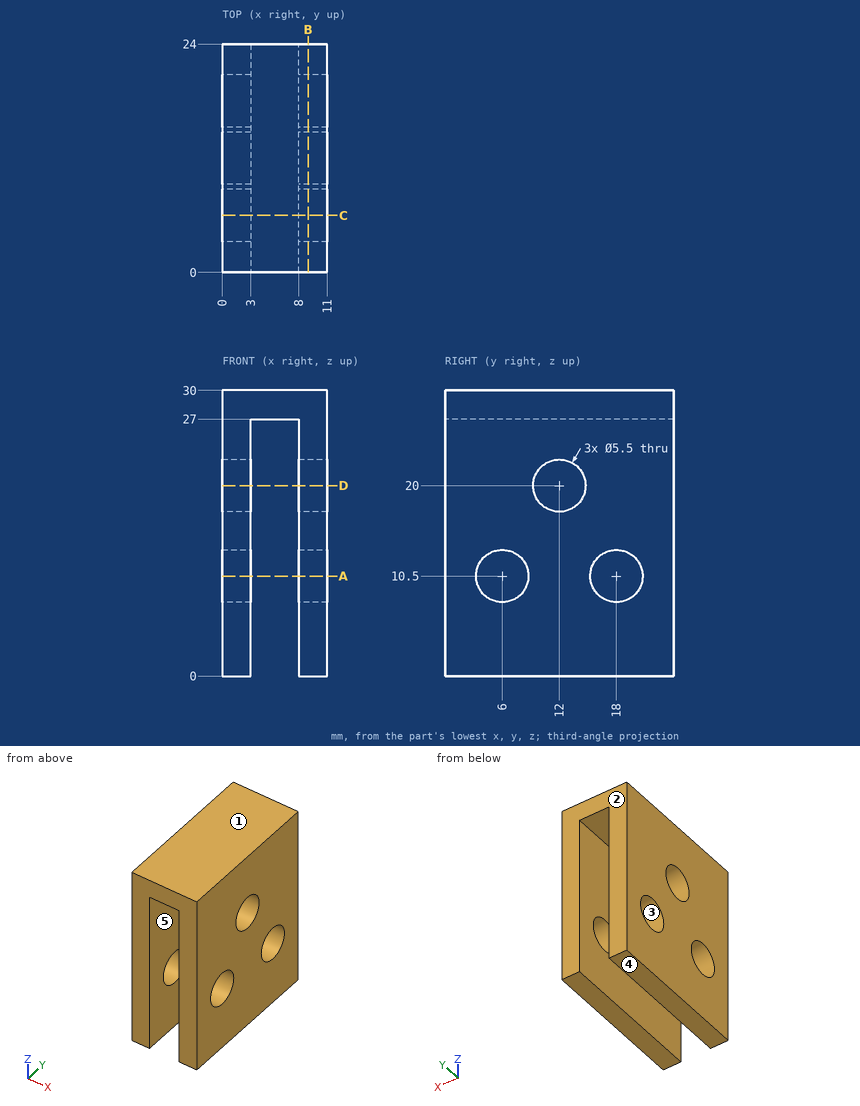
The figure shows three views and two pictorial views of one solid part (mm, origin at its lowest corner). Answer the questions. A direction names the side the tool comes from. Coordinates: 2 decimals unless noted, no trailing zeros. Loops run counter-clockwise (first coordinate to the right, second up) from the corner with the lowest first, then second, coordinate; pieces in that order, holes last.
(1) The part is cut by section B-B (x = 9). Determine the outline of the cut face in (y, z), and give its area (3 significant figures).
Solution:
outline: (0, 0) - (24, 0) - (24, 30) - (0, 30) - close; hole circle Ø5.5 at (6, 10.5); hole circle Ø5.5 at (12, 20); hole circle Ø5.5 at (18, 10.5)
area: 649 mm2
(2) The part is cut by section D-D (z = 20). Determine the outline of the cut face in (x, y).
Solution:
outline: (0, 0) - (3, 0) - (3, 9.25) - (0, 9.25) - close; (0, 14.75) - (3, 14.75) - (3, 24) - (0, 24) - close; (8, 0) - (11, 0) - (11, 9.25) - (8, 9.25) - close; (8, 14.75) - (11, 14.75) - (11, 24) - (8, 24) - close
(3) The part is cut by section A-A (z = 10.5). Determine the outline of the cut face in (x, y).
Solution:
outline: (0, 0) - (3, 0) - (3, 3.25) - (0, 3.25) - close; (0, 8.75) - (3, 8.75) - (3, 15.25) - (0, 15.25) - close; (0, 20.75) - (3, 20.75) - (3, 24) - (0, 24) - close; (8, 0) - (11, 0) - (11, 3.25) - (8, 3.25) - close; (8, 8.75) - (11, 8.75) - (11, 15.25) - (8, 15.25) - close; (8, 20.75) - (11, 20.75) - (11, 24) - (8, 24) - close
(4) Consider line 1 along Y through (x, z) = (9.05, 10.5); line 2 along X through (y, z) = (14.5, 23.5); line 3 along Y through (x, z) = (8.25, 12). Determine where each line is inside the solid, lowest interval first.
Solution:
line 1: y = 0 to 3.25, 8.75 to 15.25, 20.75 to 24
line 2: x = 0 to 3, 8 to 11
line 3: y = 0 to 3.7, 8.3 to 15.7, 20.3 to 24
(5) A tool of negligible diameter and unlimited length cuts with its end or side. For the marked faces 4 and 5, from which of +Z, -Z, +X, -X, +Y, -Y can it reach the whole face along a straight path? Write none if from no direction.
Solution:
face 4: -Z, +X, -X, +Y, -Y
face 5: -Z, +Y, -Y
(6) The part is cut by section C-C (y = 6). Determine the outline of the cut face in (x, z).
Solution:
outline: (0, 0) - (3, 0) - (3, 7.75) - (0, 7.75) - close; (0, 13.25) - (3, 13.25) - (3, 27) - (8, 27) - (8, 13.25) - (11, 13.25) - (11, 30) - (0, 30) - close; (8, 0) - (11, 0) - (11, 7.75) - (8, 7.75) - close
(7) The mould has two halves that part along Y. Classify the marked faces 1, 2 and 3: released by +Y, released by -Y, zero draft, split by the parting line, or undercut.
Solution:
face 1: zero draft
face 2: released by +Y
face 3: undercut
(8) A flat-ended cylindrical pin translates along its axis: pin 1 Ø2 at (x, y) = (6, 20) entering from -Z. Find the tip coordinate at first contact, or state that the pin passes through.
Solution:
pin 1: stops at z = 27
